from build123d import *

# Parameters (mm, degrees)
SKETCH1_R             = 6
BOSS_EXTRUDE2_DEPTH   = 7
SKETCH1_4_R           = 2
BOSS_EXTRUDE3_DEPTH   = 3
SKETCH1_5_R           = 3
CUT_EXTRUDE1_DEPTH    = 8
FILLET5_R             = 2
M3_TAPPED_HOLE2_D     = 3
M3_TAPPED_HOLE2_DEPTH = 8.5
M3_TAPPED_HOLE2_TIP   = 0.901290929


with BuildPart() as part:
    # Sketch1 → Boss-Extrude2 (new body)
    with BuildSketch(Plane.XY):
        Circle(SKETCH1_R)
    extrude(amount=BOSS_EXTRUDE2_DEPTH)

    # Sketch1<4> → Boss-Extrude3 (add)
    with BuildSketch(Plane.XY):
        with BuildLine():
            Line((3.970026899, -16.488760087), (5.820835183, -1.45529302))
            ThreePointArc((5.820835183, -1.45529302), (0, -6), (-5.820835183, -1.45529302))
            Line((-5.820835183, -1.45529302), (-3.970026899, -16.488760087))
            ThreePointArc((-3.970026899, -16.488760087), (0, -20), (3.970026899, -16.488760087))
        make_face()
        with Locations((0, -16)):
            Circle(SKETCH1_4_R, mode=Mode.SUBTRACT)
    extrude(amount=BOSS_EXTRUDE3_DEPTH)

    # Sketch1<5> → Cut-Extrude1 (cut, through all)
    with BuildSketch(Plane.XY):
        Circle(SKETCH1_5_R)
    extrude(amount=CUT_EXTRUDE1_DEPTH, mode=Mode.SUBTRACT)

    # Fillet5
    fillet5_edges = [part.edges().sort_by_distance(p)[0] for p in [
        (0, -6, 3),
    ]]
    fillet(fillet5_edges, radius=FILLET5_R)

    # M3 Tapped Hole2
    with Locations(Plane(origin=(0, 7, 0), x_dir=(1, 0, 0), z_dir=(0, 1, 0))):
        with Locations((0, -3.5)):
            Hole(M3_TAPPED_HOLE2_D / 2, depth=M3_TAPPED_HOLE2_DEPTH)
            with Locations((0, 0, -(M3_TAPPED_HOLE2_DEPTH + M3_TAPPED_HOLE2_TIP / 2))):  # 118° drill point
                Cone(0, M3_TAPPED_HOLE2_D / 2, M3_TAPPED_HOLE2_TIP, mode=Mode.SUBTRACT)


solid = part.part
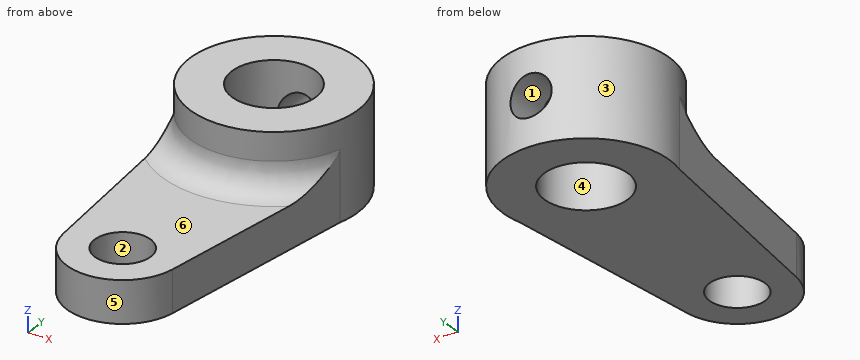
Model file for the job. Use its own axes, mm. Face numbers are marked on the shaded views. A direction names the side the tool comes from. Coordinates: 2 decimals unless noted, no trailing zeros. Loops run counter-clockwise (first coordinate to the right, second up) from the corner with the lowest first, then second, coordinate; pieces in that order, holes last. Notation, with made-up numbers: (1, 46) -> (46, 46) arc R15 ccw to (46, 56) -> close; hole circle Ø9 at (63.25, -7.5). An arc over 180 degrees is marked (long way). Use one line per item in the form item = value. Start each with the question number.
(1) Pull direction X, two halves, no side cores. Call the marked faces 4, 5 and 6: pulls with the +X half, pulls with the -X half, needs draft (parallel to the pull), parting line crosses it, or undercut.
(2) Probe probe 1 along Y at (x, z) = (0, 1.8); probe 2 along X at (y, z) = (0, 5); probe 3 along Z at (x, y) = (0, 4.9). List the from-to ranges inside material, lowest first. Write a range as from..to.
(3) Cut at A-A on x = 0. Give the cut face in (y, z), and give its area (3 significant figures).
(4) Cut at D-D on z = 1. Give the cut face in (x, y).
(5) Flat gauge pins, fed straight in: pin 1 (2 mm diameter, centred on y = -10.5, z = 5, fed in from -X); pin 2 (1.5 mm diameter, centred on y = -12, z = 1, fed in from +X) (3 decimals); pin 3 (1.5 mm diameter, centred on y = -11, z = 1, fed in from -X); pin 4 (2 mm diameter, centred on x = 3, z = 5.5, fed in from +Y). Where does each tip first touch, or does it go through?
(6) Cut at C-C on z = 2.25. Give the cut face in (x, y), and give its area (3 significant figures).
(7) Cut at B-B on y = 0. Give the cut face in (x, z).
(8) Tool access for the marked faces 1, 2 and 3: list every direction of +Z, -Z, +X, -X, +Y, -Y with a clear straight run to the whole face (end or side of a thin tool).
Values:
q1.face_4 = undercut
q1.face_5 = parting line crosses it
q1.face_6 = needs draft
q2.probe_1 = -20..-18, -14..-3, 3..6
q2.probe_2 = -6..-3, 3..6
q2.probe_3 = 0..2, 5..7
q3.outline = (-20, 0) -> (-18, 0) -> (-18, 3) -> (-20, 3) -> close; (-14, 0) -> (-3, 0) -> (-3, 7) -> (-6, 7) -> (-6, 5) arc R2 cw to (-8, 3) -> (-14, 3) -> close; (3, 0) -> (6, 0) -> (6, 2) -> (3, 2) -> close; (3, 5) -> (6, 5) -> (6, 7) -> (3, 7) -> close
q3.area = 63.9 mm2
q4.outline = (-5.82, -1.46) -> (-3.97, -16.49) arc R4 ccw to (3.97, -16.49) -> (5.82, -1.46) arc R6 ccw (long way) to start; hole circle Ø6 at (0, 0); hole circle Ø4 at (0, -16)
q5.pin_1 = through
q5.pin_2 = 4.615
q5.pin_3 = -4.74
q5.pin_4 = 5.66
q6.outline = (-5.82, -1.46) -> (-3.97, -16.49) arc R4 ccw to (3.97, -16.49) -> (5.82, -1.46) arc R6 ccw to (0.83, 5.94) -> (0.83, 2.88) arc R3 cw (long way) to (-0.83, 2.88) -> (-0.83, 5.94) arc R6 ccw to start; hole circle Ø4 at (0, -16)
q6.area = 196 mm2
q7.outline = (-6, 0) -> (-3, 0) -> (-3, 7) -> (-6, 7) -> close; (3, 0) -> (6, 0) -> (6, 7) -> (3, 7) -> close
q8.face_1 = +Y
q8.face_2 = +Z, -Z
q8.face_3 = +Z
